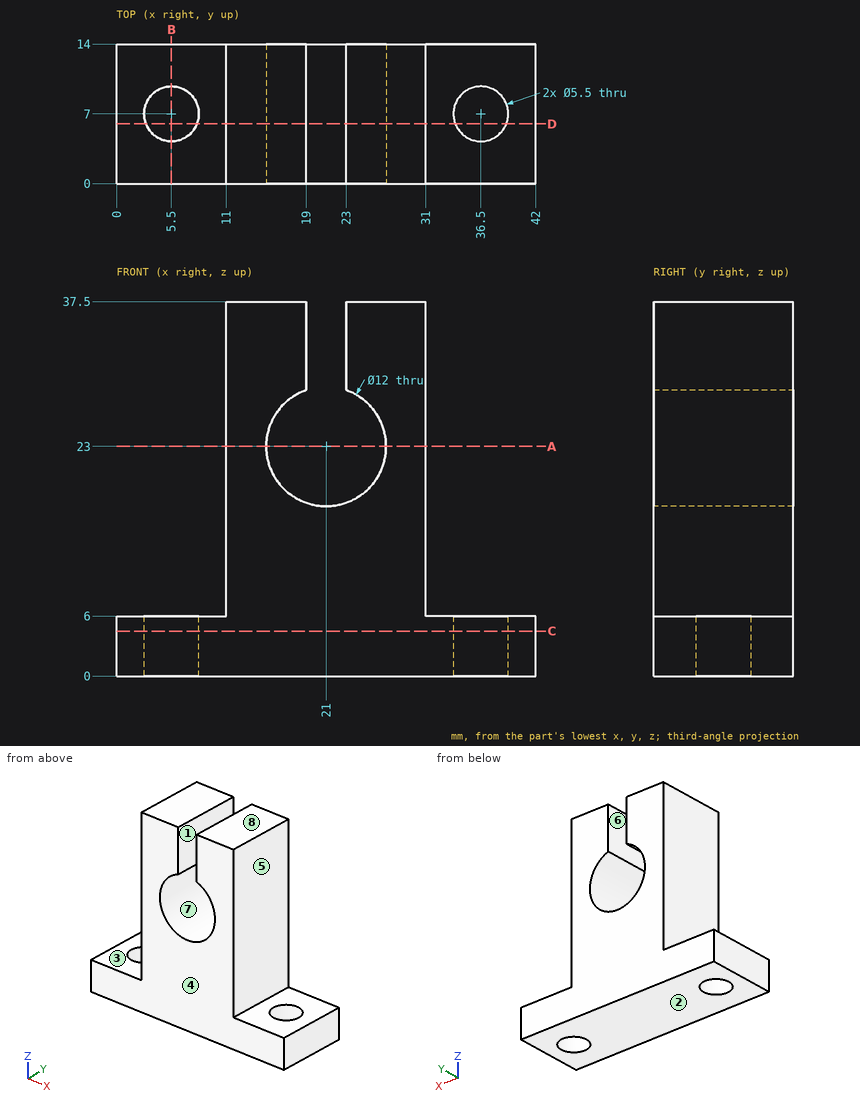
For this review, use the dimensioned drawing (mm, ordinates from the lowest corner) and the shaded views. A direction names the side the tool comes from. Coordinates: 2 decimals unless noted, no trailing zeros. Loops run counter-clockwise (first coordinate to the right, second up) from the corner with the lowest first, then second, coordinate; pieces in that order, holes last. Notation, with made-up numbers: (74, -25.5) -> (97, -25.5) arc R25 cw to (97, 13.5) -> close; hole circle Ø6 at (50.5, 53). An arc over 180 degrees is marked (long way). Return JSON: item names as keys, results as strings. Group by question number.
(1) Consider section A-A, the plane z = 23. Give the boundary of the cut face in (x, y), plus the area to 3 significant figures.
(2) Consider section D-D, the plane y = 6. Give the boundary of the cut face in (x, z), plus the area to 3 significant figures.
(3) Tool access review of the marked faces 1, 2, 3, 4 and 5: name each direction out of +Z, -Z, +X, -X, +Y, -Y from which nothing blocks a thin tool from reaching the whole face with its end or side.
(4) To check wall thickness, follow L1, parallel to X at y = 7, z = 1.5; L2, parallel to Y at x = 36.5, z = 1.8; L3, parallel to Z at x = 31.5, y = 9.25. State the ranges of each line that lie inside material, in increasing order.
(5) Mouldability with a two-part tool opening along Z and no side actions: class the marked faces 6, 7 and 8 as pulls with the +Z half, pulls with the -Z half, needs draft (parallel to the pull), parting line crosses it, or undercut.
(6) For pin 1 Ø2.5 at (y, z) = (4, 33) entering from +X, flat-tipped, find the tip position at first contact; note if it passes through.
(7) Consider section C-C, the plane z = 4.5. Give the boundary of the cut face in (x, y), plus the area to 3 significant figures.
(8) Consider section B-B, the plane x = 5.5. Give the boundary of the cut face in (y, z), plus the area to 3 significant figures.
Results below:
{
 "1": {"outline": "(11, 0) -> (15, 0) -> (15, 14) -> (11, 14) -> close; (27, 0) -> (31, 0) -> (31, 14) -> (27, 14) -> close", "area": "112 mm2"},
 "2": {"outline": "(0, 0) -> (2.94, 0) -> (2.94, 6) -> (0, 6) -> close; (8.06, 0) -> (33.94, 0) -> (33.94, 6) -> (31, 6) -> (31, 37.5) -> (23, 37.5) -> (23, 28.66) arc R6 cw (long way) to (19, 28.66) -> (19, 37.5) -> (11, 37.5) -> (11, 6) -> (8.06, 6) -> close; (39.06, 0) -> (42, 0) -> (42, 6) -> (39.06, 6) -> close", "area": "673 mm2"},
 "3": {"face 1": "+Z, +Y, -Y", "face 2": "-Z, +X, -X, +Y, -Y", "face 3": "+Z, -X, +Y, -Y", "face 4": "+Z, -Z, +X, -X, -Y", "face 5": "+Z, +X, +Y, -Y"},
 "4": {"L1": "x = 0 to 2.75, 8.25 to 33.75, 39.25 to 42", "L2": "y = 0 to 4.25, 9.75 to 14", "L3": "z = 0 to 6"},
 "5": {"face 6": "needs draft", "face 7": "undercut", "face 8": "pulls with the +Z half"},
 "6": {"pin 1": "stops at x = 31"},
 "7": {"outline": "(0, 0) -> (42, 0) -> (42, 14) -> (0, 14) -> close; hole circle Ø5.5 at (5.5, 7); hole circle Ø5.5 at (36.5, 7)", "area": "540 mm2"},
 "8": {"outline": "(0, 0) -> (4.25, 0) -> (4.25, 6) -> (0, 6) -> close; (9.75, 0) -> (14, 0) -> (14, 6) -> (9.75, 6) -> close", "area": "51.0 mm2"}
}
